Input: dimensioned drawing with shaded views. Units: mm. Origin: part minimum x, y, z. A direction names the side the tool comes from. Give positions to 0.01 mm unless a question says otherwise; leave off trailing zeros. Write each loop counter-clockwise with the first axis right and the second up, starting at its lowest first coordinate (ties: lowest second). Pieces come first, ordered by that corner, then holes.
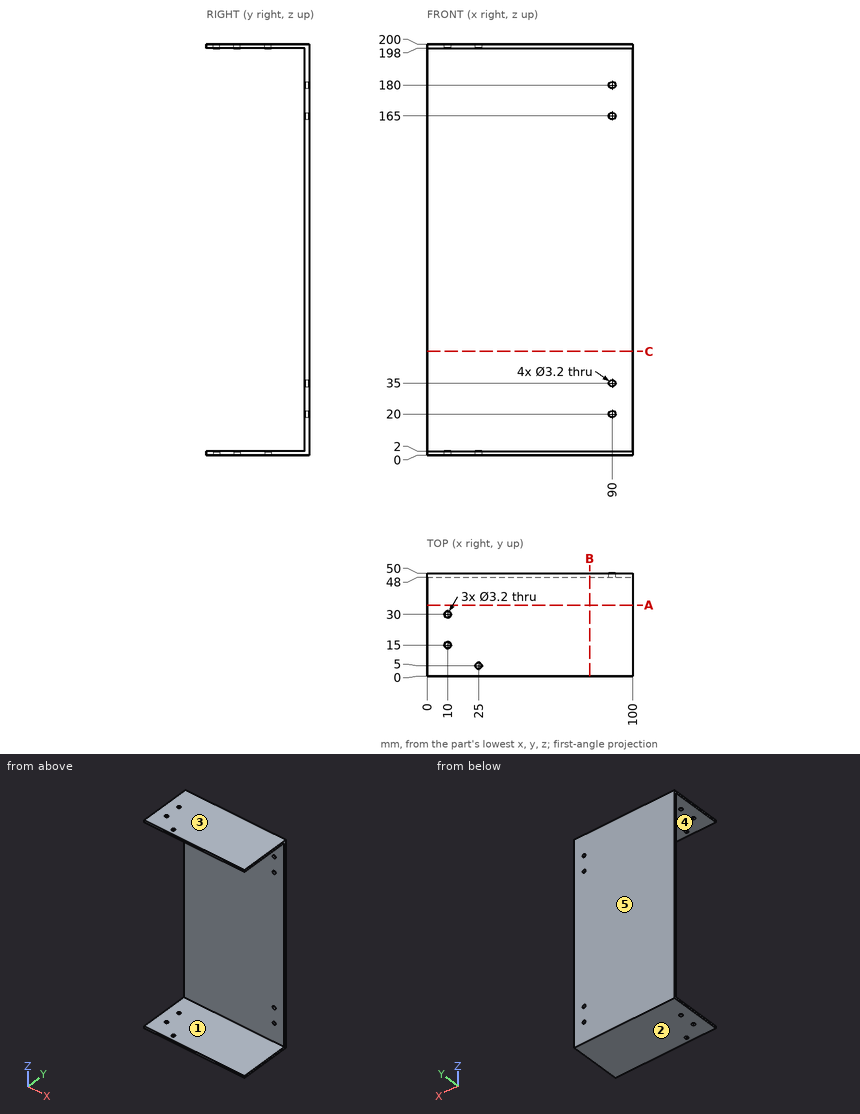
Item 1: Pin query (flat end, axial travel): pin 1 Ø4 at (x, z) = (73, 119.5) entering from -Y. Return the tip coordinate at first contact, or that it passes through.
Found:
pin 1: stops at y = 48
Item 2: Section C-C, the plane z = 50.5. Return the cut outline in (x, y), plus the area to 3 significant figures.
Found:
outline: (0, 48) - (100, 48) - (100, 50) - (0, 50) - close
area: 200 mm2
Item 3: Section A-A, the plane y = 34.5. Return the cut outline in (x, z), plus the area to 3 significant figures.
Found:
outline: (0, 0) - (100, 0) - (100, 2) - (0, 2) - close; (0, 198) - (100, 198) - (100, 200) - (0, 200) - close
area: 400 mm2
Item 4: Pull-direction query (Z, two-part tool) for the marked faces 1, 2 and 3; classes: +Z half, -Z half, draft (parallel to the pull), parting line (faces both ways), or undercut.
Found:
face 1: undercut
face 2: -Z half
face 3: +Z half
Item 5: Reachability of the marked faces 4 and 5 from +Z, -Z, +X, -X, +Y, -Y: full face, straight path, thin tool, end or side. Return the list, or none.
Found:
face 4: +X, -X, -Y
face 5: +Z, -Z, +X, -X, +Y
Item 6: Section B-B, the plane x = 79. Return the cut outline in (y, z).
Found:
outline: (0, 0) - (50, 0) - (50, 200) - (0, 200) - (0, 198) - (48, 198) - (48, 2) - (0, 2) - close
Item 7: Line query: L1, parallel to Z at x = 90, y = 49.55; L2, parallel to Z at x = 87.5, y = 13.5; L3, parallel to X at y = 48.95, z = 180. Output: solid intervals per line, ascending.
Found:
L1: z = 0 to 18.4, 21.6 to 33.4, 36.6 to 163.4, 166.6 to 178.4, 181.6 to 200
L2: z = 0 to 2, 198 to 200
L3: x = 0 to 88.4, 91.6 to 100
